Work out the finished part from the listing and answer in its coordinate system (mm). A direction names the side the tool comes from. Round coordinates to 2 decimals unless told otherwise and drop trailing zeros. Write each loop counter-clockwise with the first axis right and the second up, starting at its lowest first coordinate (ties: lowest second). Pieces come first, ordered by that corner, then holes. Notation, with made-up numbers: (-19.5, 27.5) - (-9.5, 27.5) arc R9 cw to (-9.5, 42.5) - close; hole circle Ø11 at (-8, -5.5). An arc over 180 degrees is marked (long way). Answer as a JSON object with one key per item and string values.
```python
from build123d import *

# Parameters (mm, degrees)
F0_W     = 95.491998
F0_H     = 49.64583
F0_R     = 20.059681
F1_DEPTH = 95.213123
F2_R     = 16.985566
F3_DEPTH = 65.656334


with BuildPart() as f1:
    # F0 (on Front) → F1 (new body)
    with BuildSketch(Plane.XZ):
        with Locations((12.60728, 1.098985)):
            Rectangle(F0_W, F0_H)
        with Locations((-9.042681, 0)):
            Circle(F0_R, mode=Mode.SUBTRACT)
    extrude(amount=-F1_DEPTH)

    # F2 (on face) → F3 (join)
    with BuildSketch(Plane.XY.offset(25.9219)):
        with Locations((29.532403, 45.785598)):
            Circle(F2_R)
    extrude(amount=F3_DEPTH)


solid = f1.part
```
Item 1: For faces 4 (the flat face through (23, 95.213, 1)), 5 (the cylindrical face through (16.053, 35.45, 58.29)), determine the directions among +Z, -Z, +X, -X, +Y, -Y from which every point of the face is accessible in a straight line to the end or side of a thin tool.
Results found:
{"face 4": "+Z, -Z, +X, -X, +Y", "face 5": "+Z"}
Item 2: A cutting plane is placed at C-C (y = 85). Write down the section's boundary in (x, z).
Results found:
{"outline": "(-35.14, -23.72) - (60.35, -23.72) - (60.35, 25.92) - (-35.14, 25.92) - close; hole circle Ø40.12 at (-9.04, 0)"}
Item 3: A cutting plane is placed at B-B (x = -26.5). Write down the section's boundary in (y, z).
Results found:
{"outline": "(0, -23.72) - (95.21, -23.72) - (95.21, -9.88) - (0, -9.88) - close; (0, 9.88) - (95.21, 9.88) - (95.21, 25.92) - (0, 25.92) - close"}
Item 4: Consider line 1 along Z through (x, y) = (30, 70); line 2 along X through (y, z) = (55, 13); line 3 along Z through (x, y) = (2, 10.5). Determine where each line is inside the solid, lowest interval first.
Results found:
{"line 1": "-23.72 to 25.92", "line 2": "-35.14 to -24.32, 6.23 to 60.35", "line 3": "-23.72 to -16.75, 16.75 to 25.92"}
Item 5: Determine the mould class of faces 1 (the cylindrical face through (-11.65, 46.94, 19.89)), 2 (the flat face through (-35.139, 47, 1)), 3 (the flat face through (12, 47, -23.724)) for opening direction Z: pulls with the +Z half, pulls with the -Z half, needs draft (parallel to the pull), parting line crosses it, or undercut.
Results found:
{"face 1": "undercut", "face 2": "needs draft", "face 3": "pulls with the -Z half"}
Item 6: A cutting plane is placed at A-A (z = 0). Write down the section's boundary in (x, y), and give its area (3 significant figures).
Results found:
{"outline": "(-35.14, 0) - (-29.1, 0) - (-29.1, 95.21) - (-35.14, 95.21) - close; (11.02, 0) - (60.35, 0) - (60.35, 95.21) - (11.02, 95.21) - close", "area": "5,270 mm²"}
Item 7: A cutting plane is placed at D-D (z = 66). Write down the section's boundary in (x, y).
Results found:
{"outline": "circle Ø33.97 at (29.53, 45.79)"}
Item 8: Each of these flat-tipped pins is pushed along its axis until it touches: P1, Ø4, axis at x = 14.5, y = 56.5, coming from the +Z side; P2, Ø10, axis at y = 66, z = 56.5, coming from the +X side; P3, Ø4, axis at y = 49, z = 56, coming from the +X side. Where does it stop, or does it pass through?
Results found:
{"P1": "z = 91.58", "P2": "x = 37.08", "P3": "x = 46.47"}
